```python
from build123d import *

# Parameters (mm, degrees)
F0_W     = 101.6
F0_H     = 50.8
F1_DEPTH = 76.2
F2_R     = 6.35
F3_DEPTH = 76.201
F4_W     = 25.4
F4_H     = 25.4
F6_W     = 6.35
F6_H     = 6.35
F8_R     = 5.08
F9_SIZE  = 5.08


with BuildPart() as f1:
    # F0 (on Front) → F1 (new body)
    with BuildSketch(Plane.XZ):
        Rectangle(F0_W, F0_H)
    extrude(amount=F1_DEPTH)

    # F2 (on face) → F3 (cut, through all)
    with BuildSketch(Plane.XZ.offset(76.2)):
        with Locations((-38.1, 12.7)):
            Circle(F2_R)
        with Locations((-38.1, -12.7)):
            Circle(F2_R)
        with Locations((38.1, 12.7)):
            Circle(F2_R)
        with Locations((38.1, -12.7)):
            Circle(F2_R)
    extrude(amount=-F3_DEPTH, mode=Mode.SUBTRACT)

    # F4 (on Top) → F5 (revolve)
    with BuildSketch(Plane.XY):
        with Locations((-12.7, 12.7)):
            Rectangle(F4_W, F4_H)
    revolve(axis=Axis((0, 12.7, 0), (0, -1, 0)))

    # F6 (on Top) → F7 (revolve, cut)
    with BuildSketch(Plane.XY):
        with Locations((-22.225, 15.875)):
            Rectangle(F6_W, F6_H)
    revolve(axis=Axis((0, -10.316852, 0), (0, -1, 0)), mode=Mode.SUBTRACT)

    # F8
    f8_edges = [f1.edges().sort_by_distance(p)[0] for p in [
        (25.4, 25.4, 0),
    ]]
    fillet(f8_edges, radius=F8_R)

    # F9
    f9_edges = [f1.edges().sort_by_distance(p)[0] for p in [
        (25.4, 12.7, 0),
    ]]
    chamfer(f9_edges, length=F9_SIZE)


solid = f1.part
```
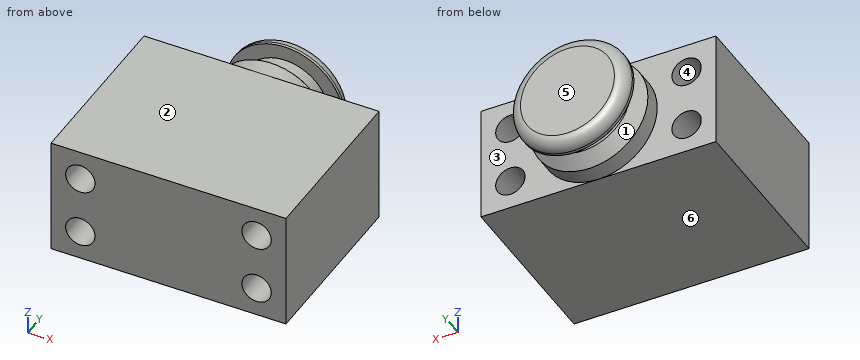
Can you work these out from the model? Positions are in its coordinate system, mm. Face numbers are marked on the shaded views. A direction names the side the tool comes from. Give positions to 0.01 mm unless a question says otherwise; leave off trailing zeros. Write each loop counter-clockwise with the first axis right and the second up, starting at its lowest first coordinate (ties: lowest second). Pieces come first, ordered by that corner, then holes. Notation, with made-up numbers: (28.25, -10.75) - (55.25, -10.75) arc R6 cw to (55.25, -2.75) - close; hole circle Ø4 at (15, -10.75). An arc over 180 degrees is marked (long way). Write item = value, one per line. Start each with the question number.
1. Please list where these lines run through material, in increasing order: line 1 (Z direction, x = -38.1, y = -36); line 2 (X direction, y = -22, z = 12); line 3 (X direction, y = -44, z = -17.5).
2. Imagine slicing it at D-D (y = 15). Please give me the cut outline in (x, z), and give its area (3 significant figures).
3. Imagine slicing it at C-C (y = -21). Please give me the cut outline in (x, z).
4. Thinking about a two-plate mould opening in Z: for the marked faces 4, 5 and 6, which applies, released by +Z, released by -Z, zero draft, split by the parting line, or undercut?
5. Imagine slicing it at A-A (x = -38.1). Please give me the cut outline in (y, z).
6. Imagine slicing it at B-B (z = 0). Please give me the cut outline in (x, y).
7. On a 3-axis mill with a long thin cutter (end or side, diameter ignored), from which of +Z, -Z, +X, -X, +Y, -Y can I reach the whole of each face in a straight line? I mean the marked faces 1, 2 and 3. Say none if no direction works.
8. For pin 1 (2 mm diameter, centred on x = 15, z = 16.5, fed in from +Y); pin 2 (16.5 mm diameter, centred on x = -38.1, z = 12.7, fed in from +Y); pin 3 (1.5 mm diameter, centred on x = -14.5, y = 3.5, fed in from +Z), each with a flat end and sliding along its axis, tell me the tip position at first contact or that it passes through.
Worked answers:
q1.line_1 = -25.4 to -19.05, -6.35 to 6.35, 19.05 to 25.4
q1.line_2 = -50.8 to -44.41, -31.79 to 31.79, 44.41 to 50.8
q1.line_3 = -50.8 to -42.26, -33.94 to 33.94, 42.26 to 50.8
q2.outline = circle Ø38.1 at (0, 0)
q2.area = 1,140 mm2
q3.outline = (-50.8, -25.4) - (50.8, -25.4) - (50.8, 25.4) - (-50.8, 25.4) - close; hole circle Ø12.7 at (-38.1, -12.7); hole circle Ø12.7 at (-38.1, 12.7); hole circle Ø12.7 at (38.1, -12.7); hole circle Ø12.7 at (38.1, 12.7)
q4.face_4 = undercut
q4.face_5 = zero draft
q4.face_6 = released by -Z
q5.outline = (-76.2, -25.4) - (0, -25.4) - (0, -19.05) - (-76.2, -19.05) - close; (-76.2, -6.35) - (0, -6.35) - (0, 6.35) - (-76.2, 6.35) - close; (-76.2, 19.05) - (0, 19.05) - (0, 25.4) - (-76.2, 25.4) - close
q6.outline = (-50.8, -76.2) - (50.8, -76.2) - (50.8, 0) - (25.4, 0) - (25.4, 7.62) - (20.32, 12.7) - (19.05, 12.7) - (19.05, 19.05) - (25.4, 19.05) - (25.4, 20.32) arc R5.08 ccw to (20.32, 25.4) - (-20.32, 25.4) arc R5.08 ccw to (-25.4, 20.32) - (-25.4, 19.05) - (-19.05, 19.05) - (-19.05, 12.7) - (-20.32, 12.7) - (-25.4, 7.62) - (-25.4, 0) - (-50.8, 0) - close
q7.face_1 = none
q7.face_2 = +Z, +X, -X, +Y, -Y
q7.face_3 = +X, +Y
q8.pin_1 = 25.3
q8.pin_2 = 0
q8.pin_3 = 21.36
